Part print with two shaded views. Sizes in mm from the minimum x, y, z corner. A direction names the side the tool comes from. Coordinates: 2 decimals unless noted, no trailing zeros. Write each loop counter-clockwise with the first axis right and the second up, starting at its lowest first coordinate (ties: lowest second). Pieces come first, ordered by that corner, then holes. Notation, with made-up numbers: (52.25, 63.25) - (75.25, 63.25) arc R29 cw to (75.25, 93.25) - close; hole circle Ø4 at (35.25, 14). An arc over 180 degrees is marked (long way). Answer in a Markdown table with one row per item. Add a question column.
Q1. Two-plate mould, pull along X, no slides. Class the marked faces 1, 2, 3 and 4: +X half, -X half, draft (parallel to the pull), parting line (faces both ways), or undercut.
Q2. Band-saw the part on D-D (z = 60). List the corners of the cut face in (x, y) (1 decimal), and give its area (3 significant figures).
Q3. Band-saw the part on A-A (y = 12). List the corners of the cut face in (x, z), and give its area (3 significant figures).
Q4. Pin check, flat tip, straight feed: pin 1 (7 mm diameter, centred on x = 111, y = 4.5, fed in from +Z). Stop position of the tip, or through.
Q5. 3-axis set-ups, long thin cutter, end or side, ignore diameter. For the marked faces 5 and 6: which of +Z, -Z, +X, -X, +Y, -Y reach the whole face in a straight line?
Q6. Band-saw the part on C-C (z = 38.5). List the corners of the cut face in (x, y) (1 decimal), and give its area (3 significant figures).
Q7. Drill centre lines: line 1 along Y through (x, z) = (61, 15) (1 decimal); line 2 along X through (y, z) = (26.5, 15); line 3 along Y through (x, z) = (11.5, 31) (1 decimal). Where is each one in solid material? Low to high. Write a range as from..to.
Q8. Band-saw the part on B-B (x = 30). List the corners of the cut face in (y, z) (1 decimal).
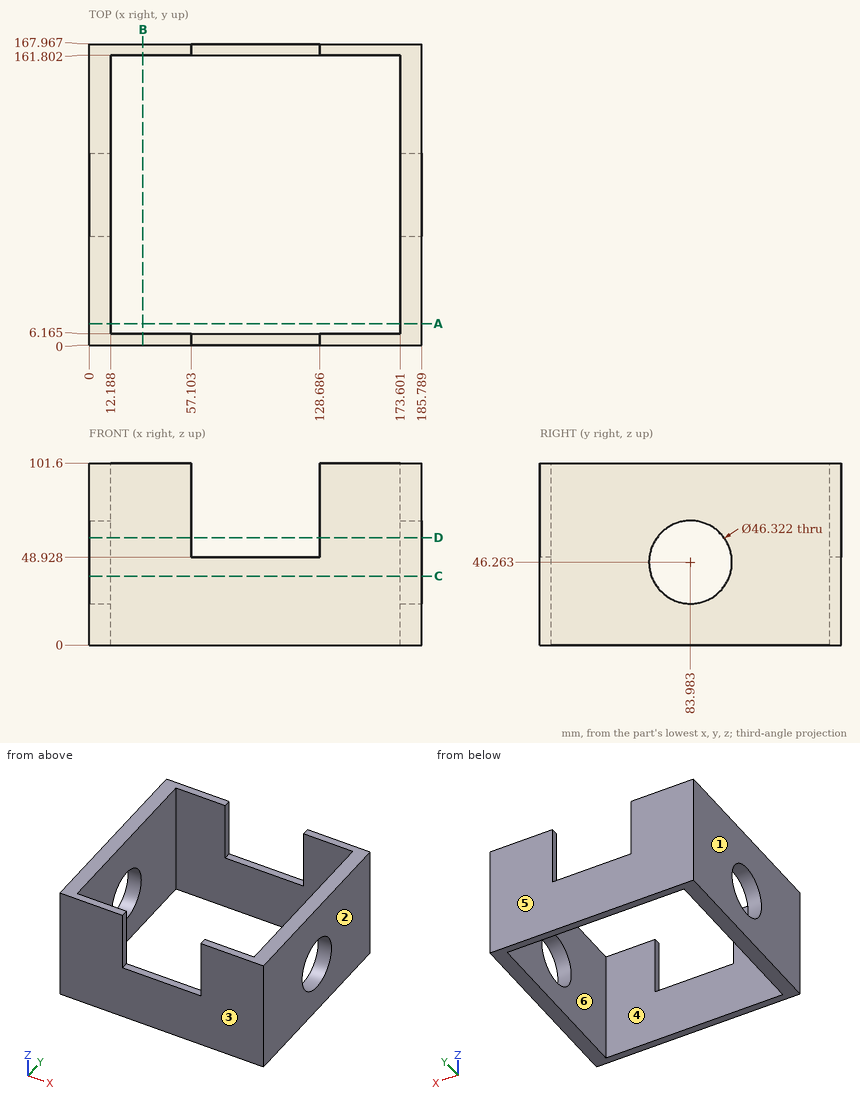
Checked values:
| question | item | result |
|---|---|---|
| 1 | face 1 | -X half |
| 1 | face 2 | +X half |
| 1 | face 3 | draft |
| 1 | face 4 | undercut |
| 2 | outline | (0, 0) - (57.1, 0) - (57.1, 6.2) - (12.2, 6.2) - (12.2, 65.3) - (0, 65.3) - close; (0, 102.6) - (12.2, 102.6) - (12.2, 161.8) - (57.1, 161.8) - (57.1, 168) - (0, 168) - close; (128.7, 0) - (185.8, 0) - (185.8, 65.3) - (173.6, 65.3) - (173.6, 6.2) - (128.7, 6.2) - close; (128.7, 161.8) - (173.6, 161.8) - (173.6, 102.6) - (185.8, 102.6) - (185.8, 168) - (128.7, 168) - close |
| 2 | area | 4,290 mm² |
| 3 | outline | (0, 0) - (12.19, 0) - (12.19, 101.6) - (0, 101.6) - close; (173.6, 0) - (185.79, 0) - (185.79, 101.6) - (173.6, 101.6) - close |
| 3 | area | 2,480 mm² |
| 4 | pin 1 | stops at z = 48.93 |
| 5 | face 5 | +Z, -Z, +X, -X, +Y |
| 5 | face 6 | +Z, -Z |
| 6 | outline | (0, 0) - (185.8, 0) - (185.8, 62.2) - (173.6, 62.2) - (173.6, 6.2) - (12.2, 6.2) - (12.2, 62.2) - (0, 62.2) - close; (0, 105.8) - (12.2, 105.8) - (12.2, 161.8) - (173.6, 161.8) - (173.6, 105.8) - (185.8, 105.8) - (185.8, 168) - (0, 168) - close |
| 6 | area | 5,020 mm² |
| 7 | line 1 | y = 0..6.2, 161.8..168 |
| 7 | line 2 | x = 0..12.19, 173.6..185.79 |
| 7 | line 3 | y = 0..66.6, 101.4..168 |
| 8 | outline | (0, 0) - (6.2, 0) - (6.2, 101.6) - (0, 101.6) - close; (161.8, 0) - (168, 0) - (168, 101.6) - (161.8, 101.6) - close |
